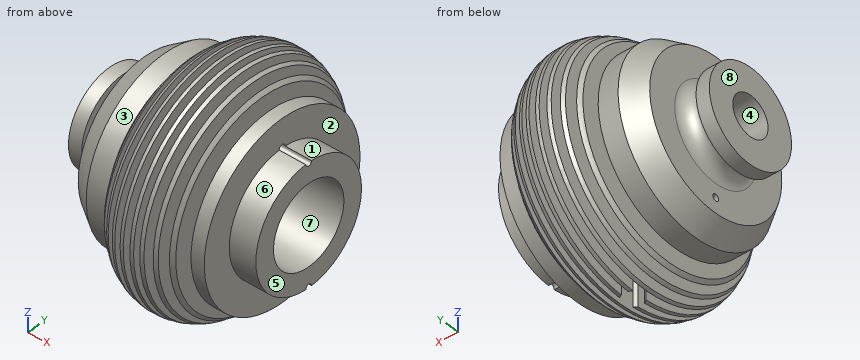
```python
from build123d import *

# Parameters (mm, degrees)
SKETCH001_R     = 7.5
POCKET_DEPTH    = 85.691761
SKETCH002_R     = 2.5
POCKET001_DEPTH = 123.858565


with BuildPart() as part:
    # Sketch → Revolution (revolve)
    with BuildSketch(Plane.XZ):
        with BuildLine():
            Line((0, 15), (50, 15))
            Line((50, 15), (50, 30))
            Line((50, 30), (150, 30))
            Line((150, 30), (150, 45))
            Line((150, 45), (130, 45))
            Line((130, 45), (130, 66.3))
            Line((130, 66.3), (120, 66.3))
            Line((120, 66.3), (120, 49.744562))
            Line((120, 49.744562), (115, 49.744562))
            Line((115, 49.744562), (115, 73.593188))
            ThreePointArc((115, 73.593188), (113.781801, 74.903585), (112.5, 76.151837))
            Line((112.5, 49.744562), (112.5, 76.151837))
            Line((112.5, 49.744562), (107.5, 49.744562))
            Line((107.5, 49.744562), (107.5, 80.026878))
            ThreePointArc((107.5, 80.026878), (106.264788, 80.786239), (105, 81.495245))
            Line((105, 49.744562), (105, 81.495245))
            Line((105, 49.744562), (100, 49.744562))
            Line((100, 49.744562), (100, 83.697181))
            ThreePointArc((100, 83.697181), (98.757097, 84.110013), (97.5, 84.477364))
            Line((97.5, 49.744562), (97.5, 84.477364))
            Line((93.565112, 49.744562), (97.5, 49.744562))
            Line((93.565112, 49.744562), (93.565112, 85.316895))
            ThreePointArc((93.565112, 85.316895), (92.317733, 85.488614), (91.065112, 85.616607))
            Line((91.065112, 49.744562), (91.065112, 85.616607))
            Line((86.065112, 49.744562), (91.065112, 49.744562))
            Line((86.065112, 49.744562), (86.065112, 85.690761))
            ThreePointArc((86.065112, 85.690761), (84.813155, 85.600321), (83.565112, 85.466292))
            Line((83.565112, 49.744562), (83.565112, 85.466292))
            Line((78.565112, 49.744562), (83.565112, 49.744562))
            Line((78.565112, 49.744562), (78.565112, 84.477364))
            ThreePointArc((78.565112, 84.477364), (77.308015, 84.110013), (76.065112, 83.697181))
            Line((76.065112, 49.744562), (76.065112, 83.697181))
            Line((71.065112, 49.744562), (76.065112, 49.744562))
            Line((71.065112, 49.744562), (71.065112, 81.495245))
            ThreePointArc((71.065112, 81.495245), (69.800323, 80.786239), (68.565112, 80.026878))
            Line((68.565112, 49.744562), (68.565112, 80.026878))
            Line((63.565112, 49.744562), (68.565112, 49.744562))
            Line((63.565112, 49.744562), (63.565112, 76.151837))
            ThreePointArc((63.565112, 76.151837), (62.283311, 74.903585), (61.065112, 73.593188))
            Line((61.065112, 49.744562), (61.065112, 73.593188))
            Line((56.065112, 49.744562), (61.065112, 49.744562))
            Line((56.065112, 66.3), (56.065112, 49.744562))
            Line((41.065112, 66.3), (56.065112, 66.3))
            Line((26.142435, 56.234528), (41.065112, 66.3))
            Line((26.142435, 34.934528), (26.142435, 56.234528))
            ThreePointArc((15, 25), (22.797345, 27.470469), (26.142435, 34.934528))
            Line((15, 25), (10, 25))
            Line((10, 25), (10, 35))
            Line((10, 35), (0, 35))
            Line((0, 35), (0, 15))
        make_face()
    revolve(axis=Axis((0, 0, 0), (1, 0, 0)))

    # Sketch001 (on DatumPlane) → Pocket (cut, through all)
    with BuildSketch(Plane(origin=(48.565112, 0, 0), x_dir=(0, 1, 0), z_dir=(0, 0, -1))):
        with Locations((0, 40)):
            Circle(SKETCH001_R)
    extrude(amount=POCKET_DEPTH, mode=Mode.SUBTRACT)

    # Sketch002 (on Face4 of Pocket) → Pocket001 (cut, through all)
    with BuildSketch(Plane(origin=(26.142435, 0, 0), x_dir=(0, 0, -1), z_dir=(-1, 0, 0))):
        with Locations((-45, 0)):
            Circle(SKETCH002_R)
        with Locations((45, 0)):
            Circle(SKETCH002_R)
    extrude(amount=-POCKET001_DEPTH, mode=Mode.SUBTRACT)


solid = part.part
```
Geometry check sheet. Reference: the model listing, model coordinates, mm. Face numbers are marked on the shaded views. A direction names the side the tool comes from. Give positions to 0.01 mm unless a question says otherwise; leave off trailing zeros. Write each loop counter-clockwise with the first axis right and the second up, starting at its lowest first coordinate (ties: lowest second). Pieces come first, ordered by that corner, then holes.
1) Section check C-C, the plane x = 140.5. Record the boundary of the cut face in (y, z).
2) Access from +Z, -Z, +X, -X, +Y, -Y to the whole of each face (thin tool, end or side, straight path). Record for the marked faces 1, 2, 3, 4 and 5.
3) Section check B-B, the plane x = 44. Record the boundary of the cut face in (y, z).
4) Release check for a two-part mould opening along Z. For the marked faces 6, 7 and 8 record: pulls with the +Z half, pulls with the -Z half, needs draft (parallel to the pull), parting line crosses it, or undercut.
5) Section check A-A, the plane y = 0. State how many separate pieces and enclosed holes the cut face has, and give its area (3 significant figures).
6) Material ranges on L1, parallel to X at y = 74, z = 29.5; L2, parallel to Z at x = 45, y = 0; L3, parallel to Y at x = 115.5, z = 0, recorded low to high.
7) Gauge pin test, flat ends, axial feed: pin 1 (12 mm diameter, centred on x = 85, z = -44, fed in from -Y); pin 2 (2 mm diameter, centred on x = 95, z = 19, fed in from +Y); pin 3 (2 mm diameter, centred on y = 0.5, z = -19, fed in from -X); pin 4 (1.5 mm diameter, centred on x = 105.5, y = 66, fed in from -Z). Record the tip position at first contact, or that the pin passes through.
Computed:
1. outline: (-2.5, -44.93) arc R2.5 cw to (2.5, -44.93) arc R45 ccw to (2.5, 44.93) arc R2.5 cw to (-2.5, 44.93) arc R45 ccw to start; hole circle Ø60 at (0, 0)
2. face 1: +X, +Y
2. face 2: +X
2. face 3: -X
2. face 4: +X, -X
2. face 5: +Z, -Z, +X, +Y, -Y
3. outline: circle Ø132.6 at (0, 0); hole circle Ø30 at (0, 0); hole circle Ø5 at (0, -45); hole circle Ø5 at (0, 45)
4. face 6: parting line crosses it
4. face 7: undercut
4. face 8: needs draft
5. separate pieces: 6
5. enclosed holes: 0
5. area: 7,080 mm2
6. L1: x = 68.57 to 71.07, 76.07 to 78.57, 83.57 to 86.07, 91.07 to 93.57, 97.5 to 100, 105 to 107.5
6. L2: z = -66.3 to -47.5, -42.5 to -15, 15 to 42.5, 47.5 to 66.3
6. L3: y = -49.74 to -30, 30 to 49.74
7. pin 1: stops at y = -76.76
7. pin 2: stops at y = 46.37
7. pin 3: stops at x = 0
7. pin 4: stops at z = -48.58
